Geometry check sheet. Reference: the model listing, model coordinates, mm. A direction names the side the tool comes from. Coordinates: 2 decimals unless noted, no trailing zeros. Order: outer loops, then holes, each group sorted by start corner. A loop starts at its lowest first (then second) coordinate and runs counter-clockwise, first axis right, second up. Notation, with made-up numbers: (80.25, -9) - (98.25, -9) arc R23 ccw to (98.25, 17) - close; hole circle Ø10 at (89, -3.5). An arc over 180 degrees is marked (long way). Put each result on its own line as item: value.
from build123d import *

# Parameters (mm, degrees)
F0_R     = 10
F0_R_2   = 5
F1_DEPTH = 5
F0_R_3   = 3
F2_DEPTH = 25
F3_R     = 5
F4_DEPTH = 5


with BuildPart() as f1:
    # F0 (on Top) → F1 (new body)
    with BuildSketch(Plane.XY):
        with Locations((-26.698679, 11.628508)):
            Circle(F0_R)
        with Locations((-26.698679, 11.628508)):
            Circle(F0_R_2, mode=Mode.SUBTRACT)
    extrude(amount=F1_DEPTH)

    # F0 (on Top) → F2 (join)
    with BuildSketch(Plane.XY):
        with Locations((-26.698679, 11.628508)):
            Circle(F0_R_2)
        with Locations((-26.698679, 11.628508)):
            Circle(F0_R_3, mode=Mode.SUBTRACT)
    extrude(amount=F2_DEPTH)

    # F3 (on face) → F4 (join)
    with BuildSketch(Plane.XY.offset(25)):
        with Locations((-26.698679, 11.628508)):
            Circle(F3_R)
    extrude(amount=F4_DEPTH)


solid = f1.part
Q1. Section check A-A on y = 14. Record the boundary of the cut face in (x, z).
Answer block:
outline: (-36.41, 0) - (-28.54, 0) - (-28.54, 25) - (-24.86, 25) - (-24.86, 0) - (-16.98, 0) - (-16.98, 5) - (-22.3, 5) - (-22.3, 30) - (-31.1, 30) - (-31.1, 5) - (-36.41, 5) - close
Q2. Thickness scan on L1, parallel to Y at x = -28.5, z = 11.75; L2, parallel to Z at x = -32.25, y = 4.75; L3, parallel to Z at x = -25.25, y = 12.5. Record the ranges inside material, lowest first. Write a range as [from, to].
Answer block:
L1: y = [6.96, 9.23], [14.03, 16.29]
L2: z = [0, 5]
L3: z = [25, 30]
Q3. Draft check along X on faces 1 (the flat face through (-29.1, 9.5, 0)), 2 (the cylindrical face through (-23.837, 12.53, 12.325)), 3 (the cylindrical face through (-27.35, 16.586, 17.325)), 4 (the flat face through (-27, 12, 25)). Enter one of: pulls with the +X half, pulls with the -X half, needs draft (parallel to the pull), parting line crosses it, or undercut.
Answer block:
face 1: needs draft
face 2: undercut
face 3: parting line crosses it
face 4: undercut
Q4. Depth check by flat-ended pin: pin 1 Ø4 at (y, z) = (7.5, 18.5) entering from -X; pin 2 Ø8 at (y, z) = (19.5, 20.5) entering from -X; pin 3 Ø2 at (x, y) = (-20.5, 14.5) entering from +Z. Enter the tip coordinate at first touch or a pass-through.
Answer block:
pin 1: stops at x = -31.22
pin 2: stops at x = -29.86
pin 3: stops at z = 5
Q5. Access from +Z, -Z, +X, -X, +Y, -Y to the whole of each face (thin tool, end or side, straight path). Record for faces 5 (the cylindrical face through (-36.69, 12.07, 2.46)), 6 (the flat face through (-31.3, 14, 5)).
Answer block:
face 5: +Z, -Z
face 6: +Z
Q6. Section check D-D on y = 8.25. Record the boundary of the cut face in (x, z), then the cut area to 3 significant figures.
Answer block:
outline: (-36.11, 0) - (-17.29, 0) - (-17.29, 5) - (-23.01, 5) - (-23.01, 30) - (-30.38, 30) - (-30.38, 5) - (-36.11, 5) - close
area: 278 mm^2
Q7. Section check B-B on z = 3. Record the boundary of the cut face in (x, y).
Answer block:
outline: circle Ø20 at (-26.7, 11.63); hole circle Ø6 at (-26.7, 11.63)
Q8. Section check C-C on x = -34.75. Record the boundary of the cut face in (y, z), then the cut area to 3 significant figures.
Answer block:
outline: (5.7, 0) - (17.56, 0) - (17.56, 5) - (5.7, 5) - close
area: 59.3 mm^2
